from build123d import *

# Parameters (mm, degrees)
SKETCH2_R           = 8.88072163
BOSS_EXTRUDE3_DEPTH = 14
SKETCH2_4_R         = 7.992649467
SKETCH2_4_R_2       = 3
BOSS_EXTRUDE4_DEPTH = 24
SKETCH2_5_R         = 7.992649467
SKETCH2_5_R_2       = 3
BOSS_EXTRUDE5_DEPTH = 6


with BuildPart() as part:
    # Sketch2 → Boss-Extrude3 (new body)
    with BuildSketch(Plane(origin=(0, 0, 0), x_dir=(1, 0, 0), z_dir=(0, 1, 0))):
        with BuildLine():
            Line((-36.813210299, 19.828534504), (-38.952982558, 20.028563155))
            ThreePointArc((-38.952982558, 20.028563155), (-50.497920677, 8.483625036), (-38.952982558, -3.061313083))
            Line((-38.952982558, -3.061313083), (-36.813210299, -2.861284433))
            ThreePointArc((-36.813210299, -2.861284433), (-30.065093762, 1.115380406), (-27.408044439, 8.483625036))
            ThreePointArc((-27.408044439, 8.483625036), (-30.065093762, 15.851869666), (-36.813210299, 19.828534504))
        make_face()
        with Locations(Location((-38.952982558, 8.483625036, 0), (0, 0, 270))):
            Circle(SKETCH2_R, mode=Mode.SUBTRACT)
    extrude(amount=BOSS_EXTRUDE3_DEPTH)



with BuildPart() as body_2:
    # Sketch2_4 → Boss-Extrude4 (new body)
    with BuildSketch(Plane(origin=(0, 0, 0), x_dir=(1, 0, 0), z_dir=(0, 1, 0))):
        with Locations(Location((-0.952982558, 8.483625036, 0), (0, 0, 270))):
            Circle(SKETCH2_4_R)
        with Locations(Location((-0.952982558, 8.483625036, 0), (0, 0, 270))):
            Circle(SKETCH2_4_R_2, mode=Mode.SUBTRACT)
    extrude(amount=-BOSS_EXTRUDE4_DEPTH)


with BuildPart() as part_1:
    add(part.part)

    add(body_2.part)  # Boss-Extrude5 merges body 2
    # Sketch2_5 → Boss-Extrude5 (add)
    # profile 1 of 2: a face of its own
    with BuildSketch(Plane(origin=(0, 0, 0), x_dir=(1, 0, 0), z_dir=(0, 1, 0))):
        with Locations(Location((-0.952982558, 8.483625036, 0), (0, 0, 270))):
            Circle(SKETCH2_5_R)
        with Locations(Location((-0.952982558, 8.483625036, 0), (0, 0, 270))):
            Circle(SKETCH2_5_R_2, mode=Mode.SUBTRACT)
    # profile 2 of 2: a face of its own
    with BuildSketch(Plane(origin=(0, 0, 0), x_dir=(1, 0, 0), z_dir=(0, 1, 0))):
        with BuildLine():
            Line((-0.952982558, 16.476274503), (-36.813210299, 19.828534504))
            ThreePointArc((-36.813210299, 19.828534504), (-30.065093762, 15.851869666), (-27.408044439, 8.483625036))
            ThreePointArc((-27.408044439, 8.483625036), (-30.065093762, 1.115380406), (-36.813210299, -2.861284433))
            Line((-36.813210299, -2.861284433), (-0.952982558, 0.490975569))
            ThreePointArc((-0.952982558, 0.490975569), (-8.945632025, 8.483625036), (-0.952982558, 16.476274503))
        make_face()
    extrude(amount=BOSS_EXTRUDE5_DEPTH)


solid = part_1.part
Source: CAD feature listing. Evaluate the final solid. Frame: model axes, mm. Round coordinates to 2 decimals unless told otherwise and drop trailing zeros. Order: outer loops, then holes, each group sorted by start corner. A loop starts at its lowest first (then second) coordinate and runs counter-clockwise, first axis right, second up. Notation, with made-up numbers: (79.25, 68.25) - (121.25, 68.25) arc R27 cw to (121.25, 85.25) - close; hole circle Ø4 at (45.25, 78). An arc over 180 degrees is marked (long way). Use a Markdown table: item, result. Add a question column.
1. Section query B-B (y = 10.5). Return the cut outline in (x, z).
2. Section query D-D (z = -2.25). Return the cut outline in (x, y).
3. First-contact query: pin 1 (12 mm diameter, centred on x = -2.5, y = 7, fed in from +Z); pin 2 (2 mm diameter, centred on x = -20, z = -9.5, fed in from -Y); pin 3 (4 mm diameter, centred on x = -1.5, z = -11.5, fed in from +Y). Flat tips, straight axial feed; report the tip coordinate or a pass-through.
4. Line query: probe 1 along Y at (x, z) = (-14.5, -2.25); probe 2 along Z at (x, y) = (1.5, -3); probe 3 along X at (y, z) = (-2.5, -8.5). Output: solid intervals per line, ascending.
5. Mould query, pull axis Z, two halves, no side actions, for faces 1 (the flat face through (-35.6, 14, 0)), 2 (the cylindrical face through (-0.052, -9.21, -5.622)), 3 (the cylindrical face through (6.972, -9.21, -9.524)). Classes: +Z half, -Z half, draft (parallel to the pull), parting line (faces both ways), or undercut.
6. Section query A-A (x = -2). Return the cut outline in (y, z).
7. Section query C-C (z = -10.75). Return the cut outline in (x, y), then the cut area to 3 significant figures.
Derived:
| question | item | result |
|---|---|---|
| 1 | outline | (-38.95, -20.03) - (-36.81, -19.83) arc R11.54 ccw to (-36.81, 2.86) - (-38.95, 3.06) arc R11.54 ccw to start; hole circle Ø17.76 at (-38.95, -8.48) |
| 2 | outline | (-48.67, 0) - (-45.28, 0) - (-45.28, 14) - (-48.67, 14) - close; (-32.63, 0) - (-5.96, 0) - (-5.96, -24) - (4.05, -24) - (4.05, 6) - (-29.24, 6) - (-29.24, 14) - (-32.63, 14) - close |
| 3 | pin 1 | z = 0.21 |
| 3 | pin 2 | y = 0 |
| 3 | pin 3 | y = 6 |
| 4 | probe 1 | 0 to 6 |
| 4 | probe 2 | -16.09 to -10.21, -6.76 to -0.88 |
| 4 | probe 3 | -8.95 to -3.95, 2.05 to 7.04 |
| 5 | face 1 | draft |
| 5 | face 2 | undercut |
| 5 | face 3 | parting line |
| 6 | outline | (-24, -16.41) - (0, -16.41) - (0, -16.57) - (6, -16.57) - (6, -11.29) - (-24, -11.29) - close; (-24, -5.67) - (6, -5.67) - (6, -0.39) - (0, -0.39) - (0, -0.56) - (-24, -0.56) - close |
| 7 | outline | (-50.27, 0) - (-47.54, 0) - (-47.54, 14) - (-50.27, 14) - close; (-30.37, 0) - (-8.62, 0) - (-8.62, -24) - (-2.92, -24) - (-2.92, 6) - (-27.63, 6) - (-27.63, 14) - (-30.37, 14) - close; (1.01, -24) - (6.71, -24) - (6.71, 6) - (1.01, 6) - close |
| 7 | area | 533 mm2 |
